Input: part model. Units: mm. Frame: model coordinates. Give positions to 0.01 mm unless a question says otherwise; leave off trailing zeros. Loops run counter-clockwise (first coordinate to the right, second up) from the corner with the lowest first, then second, coordinate; pieces in that order, holes last. Notation, with made-up numbers: (5, -34.75) - (24, -34.75) arc R18 ccw to (24, -24.75) - close; hole circle Ø11 at (11.25, -1). An arc over 180 degrees is marked (long way). Answer as a JSON object with one key per item and string values.
from build123d import *

# Parameters (mm, degrees)
F1_DEPTH = 25.4


with BuildPart() as f1:
    # F0 (on Front) → F1 (new body)
    with BuildSketch(Plane.XZ):
        with BuildLine():
            ThreePointArc((-96.2938510095, 49.8640834202), (-106.1566639379, 55.4102805892), (-117.4718999148, 55.3817029315))
            ThreePointArc((-117.4718999148, 55.3817029315), (-130.9864974324, 45.0518805264), (-133.238473511, 28.1913295056))
            ThreePointArc((-133.238473511, 28.1913295056), (-111.9975569081, 11.6794990469), (-90.4085331471, 27.7335059074))
            Line((-90.4085331471, 27.7335059074), (-96.2938510095, 49.8640834202))
        make_face()
        with BuildLine():
            Line((-99.0630919931, 60.2772681748), (-117.4718999148, 55.3817029315))
            ThreePointArc((-117.4718999148, 55.3817029315), (-106.1566639379, 55.4102805892), (-96.2938510095, 49.8640834202))
            Line((-96.2938510095, 49.8640834202), (-99.0630919931, 60.2772681748))
        make_face()
        with BuildLine():
            ThreePointArc((-90.4085331471, 27.7335059074), (-111.9975569081, 11.6794990469), (-133.238473511, 28.1913295056))
            Line((-133.238473511, 28.1913295056), (-106.1467650121, -73.6816990901))
            ThreePointArc((-106.1467650121, -73.6816990901), (-92.8623116551, -53.860643351), (-74.9299982186, -69.6017705795))
            ThreePointArc((-74.9299982186, -69.6017705795), (-79.5796780672, -80.8270907309), (-90.8049982186, -85.4767705795))
            Line((-90.8049982186, -85.4767705795), (-20.9549982186, -85.4767705795))
            ThreePointArc((-20.9549982186, -85.4767705795), (-32.1803231924, -58.3764516879), (-5.0800017814, -69.6017705795))
            ThreePointArc((-5.0800017814, -69.6017705795), (-5.2138745529, -71.659084016), (-5.6132349879, -73.6816990901))
            Line((-5.6132349879, -73.6816990901), (21.478473511, 28.1913295056))
            ThreePointArc((21.478473511, 28.1913295056), (0.2375569081, 11.6794990469), (-21.3514668529, 27.7335059074))
            Line((-21.3514668529, 27.7335059074), (-34.401526489, -21.3386704944))
            ThreePointArc((-34.401526489, -21.3386704944), (-55.88, -37.8517705795), (-77.358473511, -21.3386704944))
            Line((-77.358473511, -21.3386704944), (-90.4085331471, 27.7335059074))
        make_face()
        with BuildLine():
            ThreePointArc((-74.9299982186, -69.6017705795), (-92.8623116551, -53.860643351), (-106.1467650121, -73.6816990901))
            ThreePointArc((-106.1467650121, -73.6816990901), (-100.4809157434, -82.1871686683), (-90.8049982186, -85.4767705795))
            ThreePointArc((-90.8049982186, -85.4767705795), (-79.5796780672, -80.8270907309), (-74.9299982186, -69.6017705795))
        make_face()
        with BuildLine():
            ThreePointArc((-5.0800017814, -69.6017705795), (-32.1803231924, -58.3764516879), (-20.9549982186, -85.4767705795))
            ThreePointArc((-20.9549982186, -85.4767705795), (-11.2790828443, -82.1871675825), (-5.6132349879, -73.6816990901))
            ThreePointArc((-5.6132349879, -73.6816990901), (-5.2138745529, -71.659084016), (-5.0800017814, -69.6017705795))
        make_face()
        with BuildLine():
            Line((-15.4661489905, 49.8640834202), (-21.3514668529, 27.7335059074))
            ThreePointArc((-21.3514668529, 27.7335059074), (0.2375569081, 11.6794990469), (21.478473511, 28.1913295056))
            ThreePointArc((21.478473511, 28.1913295056), (22.0375781199, 31.0229906094), (22.225, 33.9032294205))
            ThreePointArc((22.225, 33.9032294205), (17.6195573243, 47.4495139552), (5.7118999148, 55.3817029315))
            ThreePointArc((5.7118999148, 55.3817029315), (-5.6033360621, 55.4102805892), (-15.4661489905, 49.8640834202))
        make_face()
        with BuildLine():
            Line((-12.6969080069, 60.2772681748), (-15.4661489905, 49.8640834202))
            ThreePointArc((-15.4661489905, 49.8640834202), (-5.6033360621, 55.4102805892), (5.7118999148, 55.3817029315))
            Line((5.7118999148, 55.3817029315), (-12.6969080069, 60.2772681748))
        make_face()
    extrude(amount=F1_DEPTH)


solid = f1.part
Item 1: Material intervals for line 1 (X direction, y = -11, z = 1.5); line 2 (X direction, y = -1.75, z = 45); line 3 (X direction, y = -21.5, z = -44), sorted ascending. Write a range as [from, to].
Geometry check:
{"line 1": "x = [-126.14, -83.43], [-28.33, 14.38]", "line 2": "x = [-131.02, -95], [-16.76, 19.26]", "line 3": "x = [-114.04, 2.28]"}
Item 2: Cut plane C-C (z = -35). Return loops of the section in (x, y), then the cut area to 3 significant figures.
Geometry check:
{"outline": "(-116.43, -25.4) - (-66.77, -25.4) - (-66.77, 0) - (-116.43, 0) - close; (-44.99, -25.4) - (4.67, -25.4) - (4.67, 0) - (-44.99, 0) - close", "area": "2,520 mm2"}
Item 3: Mould query, pull axis X, two halves, no side actions, for faces 1 (the face through (-130.863, -12.522, 45.263)), 2 (the face through (7.743, -12.522, -23.458)), 3 (the face through (-55.472, -12.522, -37.848)). Classes: released by +X, released by -X, zero draft, split by the parting line, or undercut.
Geometry check:
{"face 1": "released by -X", "face 2": "released by +X", "face 3": "undercut"}
Item 4: Cut plane B-B (y = -21.25). Return loops of the section in (x, z) (3 decimals).
Geometry check:
{"outline": "(-133.238, 28.191) - (-106.147, -73.682) arc R15.875 ccw to (-90.805, -85.477) - (-20.955, -85.477) arc R15.875 ccw to (-5.613, -73.682) - (21.478, 28.191) arc R22.225 ccw to (5.712, 55.382) - (-12.697, 60.277) - (-34.402, -21.339) arc R22.225 cw to (-77.358, -21.339) - (-99.063, 60.277) - (-117.472, 55.382) arc R22.225 ccw to start"}
Item 5: Cut plane D-D (x = -101.5). Return loops of the section in (y, z), then the cut area to 3 significant figures.
Geometry check:
{"outline": "(-25.4, -81.33) - (0, -81.33) - (0, 59.63) - (-25.4, 59.63) - close", "area": "3,580 mm2"}
Item 6: Contact query for flat-ended pins moving along their axis: P1, Ø5, axis at y = -11, z = -60, coming from the +X side; P2, Ø8, axis at y = -19, z = 44, coming from the +X side; P3, Ø8, axis at y = -7, z = -21, coming from the +X side. Output: stop coordinate, or through.
Geometry check:
{"P1": "stops at x = -1.31", "P2": "stops at x = 21.37", "P3": "stops at x = 9.46"}
Item 7: Cut plane A-A (z = 11.5). Return loops of the section in (x, y).
Geometry check:
{"outline": "(-128.8, -25.4) - (-86.09, -25.4) - (-86.09, 0) - (-128.8, 0) - close; (-25.67, -25.4) - (17.04, -25.4) - (17.04, 0) - (-25.67, 0) - close"}
